from build123d import *

# Parameters (mm, degrees)
F0_R     = 4
F0_R_2   = 1.2
F1_DEPTH = 4.2
F4_SIZE  = 0.4
F2_R     = 4
F2_R_2   = 3
F3_DEPTH = 4.2


with BuildPart() as f1:
    # F0 (on Top) → F1 (new body)
    with BuildSketch(Plane.XY):
        Circle(F0_R)
        Circle(F0_R_2, mode=Mode.SUBTRACT)
    extrude(amount=F1_DEPTH)

    # F4
    f4_edges = [f1.edges().sort_by_distance(p)[0] for p in [
        (-1.2, 0, 0),
    ]]
    chamfer(f4_edges, length=F4_SIZE)

    # F2 (on face) → F3 (join)
    with BuildSketch(Plane.XY.offset(4.2)):
        Circle(F2_R)
        Circle(F2_R_2, mode=Mode.SUBTRACT)
    extrude(amount=F3_DEPTH)


solid = f1.part
Verification items for the finished model (mm, model axes). A direction names the side the tool comes from. Coordinates: 2 decimals unless noted, no trailing zeros. Write each loop counter-clockwise with the first axis right and the second up, starting at its lowest first coordinate (ties: lowest second). Pieces come first, ordered by that corner, then holes. Notation, with made-up numbers: M -14,87.25 L 22,87.25 A9 ccw 22,98.25 Z; hole C -32.75,30.25 d6. An arc over 180 degrees is marked long. One line per question, with ' | ' between items.
1) Access from +Z, -Z, +X, -X, +Y, -Y to the whole of each face (thin tool, end or side, straight path). Record for faces 4 (the face through (1, -1, 4.2)), 5 (the face through (1, 3, 8.4)).
Solutions:
face 4: +Z | face 5: +Z, +X, -X, +Y, -Y
2) Material ranges on L1, parallel to Y at x = 0, z = 1.95; L2, parallel to Y at x = 0, z = 6.5; L3, parallel to Z at x = 1.25, y = 1.25, recorded low to high.
Solutions:
L1: -4 to -1.2, 1.2 to 4 | L2: -4 to -3, 3 to 4 | L3: 0 to 4.2
3) Depth check by flat-ended pin: pin 1 Ø3 at (x, y) = (-1.5, 1) entering from +Z; pin 2 Ø4 at (x, z) = (3, 1.5) entering from +Y; pin 3 Ø4 at (x, y) = (0, 0) entering from +Z; pin 4 Ø2 at (y, z) = (2, 3) entering from +X. Enter the tip coordinate at first touch or a pass-through.
Solutions:
pin 1: z = 8.4 | pin 2: y = 3.87 | pin 3: z = 4.2 | pin 4: x = 3.87
4) Sectioned sample at D-D on x = 2.5. Record the cut outline in (y, z).
Solutions:
outline: M -3.12,0 L 3.12,0 L 3.12,8.4 L 1.66,8.4 L 1.66,4.2 L -1.66,4.2 L -1.66,8.4 L -3.12,8.4 Z
5) Release check for a two-part mould opening along Y. For faces 1 (the face through (0.65, 1.01, 2.27)), 2 (the face through (-0.867, -3.905, 4.141)), 3 (the face through (2, 0, 0)) record: +Y half, -Y half, draft (parallel to the pull), parting line (faces both ways), or undercut.
Solutions:
face 1: undercut | face 2: parting line | face 3: draft
6) Sectioned sample at A-A on y = 0. Record the cut outline in (x, z).
Solutions:
outline: M -4,0 L -1.6,0 L -1.2,0.4 L -1.2,4.2 L -3,4.2 L -3,8.4 L -4,8.4 Z; M 1.2,0.4 L 1.6,0 L 4,0 L 4,8.4 L 3,8.4 L 3,4.2 L 1.2,4.2 Z
7) Sectioned sample at C-C on z = 4. Record the cut outline in (x, y), then the cut area to 3 significant figures.
Solutions:
outline: C 0,0 d8; hole C 0,0 d2.4 | area: 45.7 mm^2
